from build123d import *

# Parameters (mm, degrees)
SKETCH1_R           = 3.2639
BOSS_EXTRUDE1_DEPTH = 3.175
CAVITY1_START       = 3.689049998
CAVITY1_DEPTH       = 9.603434939
FILLET3_R           = 1.27


# Read off the part's stored shape, not the designer's step: Cavity1
with BuildPart() as part:
    # Sketch1 → Boss-Extrude1 (new body)
    with BuildSketch(Plane.XY):
        with BuildLine():
            ThreePointArc((9.406966983, 1.494856913), (0, 9.525), (-9.406966983, 1.494856913))
            Line((-9.406966983, 1.494856913), (-15.24, -35.211766))
            Line((-15.24, -35.211766), (15.24, -35.211766))
            Line((15.24, -35.211766), (9.406966983, 1.494856913))
        make_face()
        Circle(SKETCH1_R, mode=Mode.SUBTRACT)
    extrude(amount=BOSS_EXTRUDE1_DEPTH)

    # Cavity1 outline → Cavity1 (cut)
    with BuildSketch(Plane(origin=(0, 0, 0), x_dir=(0.9955947349362284, 0.032256539947670526, 0.08803771576924041), z_dir=(0.09376099278090663, -0.3425138790307331, -0.9348225066311033)).offset(CAVITY1_START)):
        with BuildLine():
            Line((-14.012226084, 36), (-14.169183947, 34.154693399))
            ThreePointArc((-14.169183947, 34.154693399), (-1.135248211, 19.965054491), (11.898687525, 34.154693399))
            Line((11.898687525, 34.154693399), (11.741729662, 36))
            Line((11.741729662, 36), (-14.012226084, 36))
        make_face()
    extrude(amount=CAVITY1_DEPTH, mode=Mode.SUBTRACT)

    # Fillet3
    fillet3_edges = [part.edges().sort_by_distance(p)[0] for p in [
        (-15.24, -35.211766, 1.5875),
        (15.24, -35.211766, 1.5875),
    ]]
    fillet(fillet3_edges, radius=FILLET3_R)


solid = part.part
Work out the finished part from the listing and answer in its coordinate system (mm). Give positions to 0.01 mm unless a question says otherwise; leave off trailing zeros. Loops run counter-clockwise (first coordinate to the right, second up) from the corner with the lowest first, then second, coordinate; pieces in that order, holes last. Notation, with made-up numbers: M 11,-15 L 36,-15 A34 cw 36,16 Z; hole C -3,74 d1. An arc over 180 degrees is marked long. Use CSV: the item, a comma, the result in double quotes.
1) Determine the mould class of faces 1 (the cylindrical face through (14.73, -34.75, 1.61)), 2 (the cylindrical face through (-0.708, -3.186, 1.565)), 3 (the flat face through (-12.17, -15.88, 1.57)) for opening direction X: released by +X, released by -X, zero draft, split by the parting line, or undercut.
Answer:
face 1,"released by +X"
face 2,"undercut"
face 3,"released by -X"
2) Find section B-B on y = -12. Write down the section's boundary in (x, z) (3 decimals), plus the area to 3 significant figures.
Answer:
outline,"M -11.551,0 L 11.551,0 L 11.551,3.175 L -11.551,3.175 Z"
area,"73.4 mm^2"
3) Find section A-A on y = 0. Write down the section's boundary in (x, z) (3 decimals).
Answer:
outline,"M -9.645,0 L -3.264,0 L -3.264,3.175 L -9.645,3.175 Z; M 3.264,0 L 9.645,0 L 9.645,3.175 L 3.264,3.175 Z"
4) Find section C-C on y = -6.5. Write down the section's boundary in (x, z) (3 decimals).
Answer:
outline,"M -10.677,0 L 10.677,0 L 10.677,3.175 L -10.677,3.175 Z"
5) Consider L1, parallel to Y at x = 0, z = 1.2 (3 decimals); L2, parallel to X at y = -24, z = 2.05; L3, parallel to Y at x = 0, z = 0.7 (3 decimals). Determine where each line is inside the solid, lowest interval first.
Answer:
L1,"-20.836 to -3.264, 3.264 to 9.525"
L2,"-13.46 to -9.24, 8.15 to 13.46"
L3,"-21.017 to -3.264, 3.264 to 9.525"
6) Given P1, Ø1.5, axis at y = -30.5, z = 1, coming from the +X side, flat-ended and moving along its own axis, determine where the tip first touches the part or whether it passes through.
Answer:
P1,"x = 14.61"
